The drawing under review shows one solid part. Ordinate dimensions are in mm from its lowest x, y, z. A direction names the side the tool comes from. Coordinates: 2 decimals unless noted, no trailing zeros. Write each loop counter-clockwise with the first axis right and the second up, starting at its lowest first coordinate (ties: lowest second). Pieces come first, ordered by that corner, then holes. Notation, with made-up numbers: (80, 4.5) -> (102, 4.5) arc R31 cw to (102, 33.5) -> close; hole circle Ø6 at (72.25, -23). An arc over 180 degrees is marked (long way). One line per question, with ' | ' between items. Start each with the question number.
Q1. Add section C-C on x = 57.15. State the section outline as (y, z) points (3 decimals).
Q2. Draft analysis for pull direction X (two halves, no side actions). For the marked faces 1, 2, 3 and 4, state which applies: pulls with the +X half, pulls with the -X half, needs draft (parallel to the pull), parting line crosses it, or undercut.
Q3. For P1, Ø8, axis at x = 24, z = 13, coming from the -Y side; P2, Ø1, axis at y = 23.5, z = 1, coming from the +X side; P3, Ø1.5, axis at x = 56.5, z = 0.5, coming from the +Y side; P4, Ø3, axis at y = 45.5, z = 7, coming from the +X side (3 decimals), all flat-tipped, find the tip position at first contact; note any pin that passes through.
Q4. Add section D-D on z = 7. Give the number of separate pieces and of enclosed holes in the cut face, and give its area (3 significant figures).
Q5. For the marked faces 5, 6, 7 and 8, list the 3-axis set-ups (+Z, -Z, +X, -X, +Y, -Y) from which the entire face can be reached by the end or side of a thin tool; tool diameter is ignored.
Q6. Wall thickness on probe 1 along Y at (x, z) = (57.15, 15); probe 2 along X at (y, z) = (63.5, 4) (3 decimals); probe 3 along Y at (x, z) = (67, 9.5): over which ranges is each line inside the solid? List them lowest first.
Q7. Add section B-B on y = 26.5. State the section outline as (x, z) points (3 decimals).
Q8. Add section A-A on y = 52.55. State the section outline as (x, z) points (3 decimals).
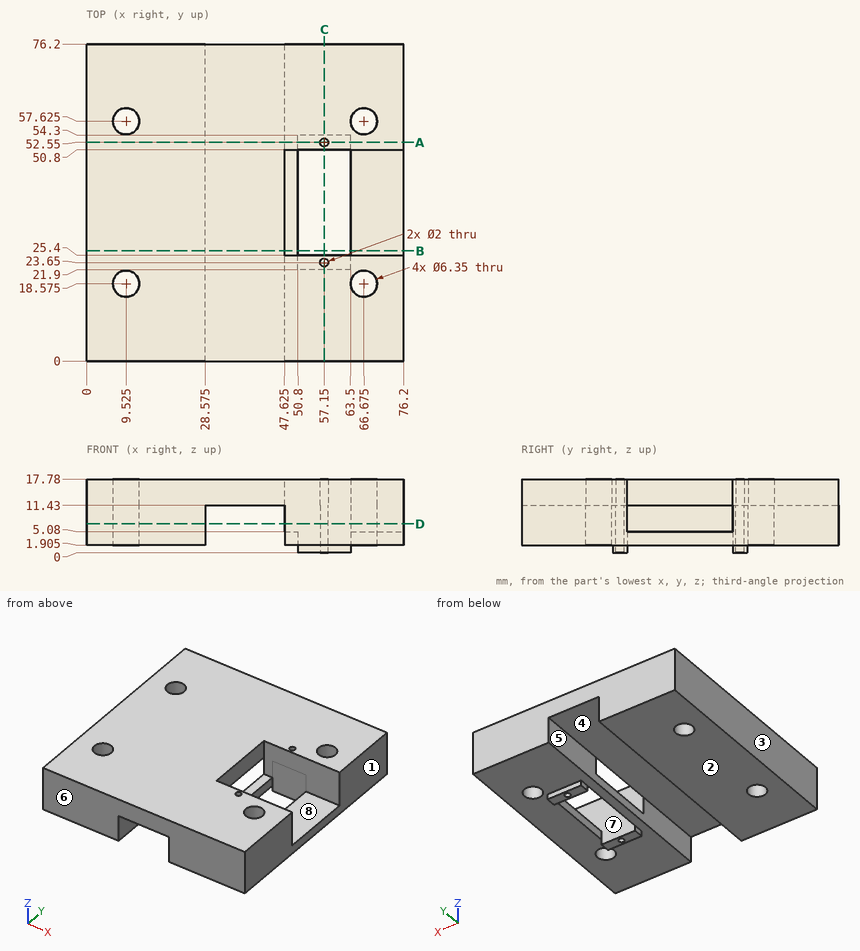
Output values:
1) outline: (0, 1.905) -> (21.9, 1.905) -> (21.9, 0) -> (22.65, 0) -> (22.65, 17.78) -> (0, 17.78) -> close; (24.65, 0) -> (25.4, 0) -> (25.4, 17.78) -> (24.65, 17.78) -> close; (50.8, 0) -> (51.55, 0) -> (51.55, 17.78) -> (50.8, 17.78) -> close; (53.55, 0) -> (54.3, 0) -> (54.3, 1.905) -> (76.2, 1.905) -> (76.2, 17.78) -> (53.55, 17.78) -> close
2) face 1: pulls with the +X half | face 2: needs draft | face 3: pulls with the -X half | face 4: undercut
3) P1: stops at y = 0 | P2: stops at x = 63.5 | P3: stops at y = 54.3 | P4: stops at x = 28.575
4) separate pieces: 3 | enclosed holes: 6 | area: 3,500 mm2
5) face 5: -Z, +Y, -Y | face 6: +Z, -Z, +X, -X, -Y | face 7: +Z | face 8: +Z, +X
6) probe 1: y = 0 to 22.65, 24.65 to 25.4, 50.8 to 51.55, 53.55 to 76.2 | probe 2: x = 0 to 28.575, 47.625 to 76.2 | probe 3: y = 0 to 15.42, 21.73 to 25.4, 50.8 to 54.47, 60.78 to 76.2
7) outline: (0, 1.905) -> (28.575, 1.905) -> (28.575, 11.43) -> (47.625, 11.43) -> (47.625, 17.78) -> (0, 17.78) -> close; (47.625, 1.905) -> (50.8, 1.905) -> (50.8, 5.08) -> (47.625, 5.08) -> close; (63.5, 1.905) -> (76.2, 1.905) -> (76.2, 5.08) -> (63.5, 5.08) -> close
8) outline: (0, 1.905) -> (28.575, 1.905) -> (28.575, 11.43) -> (47.625, 11.43) -> (47.625, 1.905) -> (50.8, 1.905) -> (50.8, 0) -> (56.15, 0) -> (56.15, 17.78) -> (0, 17.78) -> close; (58.15, 0) -> (63.5, 0) -> (63.5, 1.905) -> (76.2, 1.905) -> (76.2, 17.78) -> (58.15, 17.78) -> close
